Autodesk Inventor part; units mm, degrees
ref_plane "YZ Plane" through (0, 0, 0) normal (1, 0, 0) x (0, 1, 0)
ref_plane "XZ Plane" through (0, 0, 0) normal (0, 1, 0) x (-1, 0, 0)
ref_plane "XY Plane" through (0, 0, 0) normal (0, 0, 1) x (1, 0, 0)
sketch "スケッチ1" plane through (0, 0, 0) normal (0, 0, 1) x (1, 0, 0)
  line L0 (-25, -20) -> (25, -20)
  line L1 (25, -20) -> (25, 20)
  line L2 (25, 20) -> (-25, 20)
  line L3 (-25, 20) -> (-25, -20)
  line L4 (-25, -20) -> (25, 20) construction
  line L5 (25, -20) -> (-25, 20) construction
  line L6 (-22, -17) -> (22, -17) construction
  line L7 (22, -17) -> (22, 17) construction
  line L8 (22, 17) -> (-22, 17) construction
  line L9 (-22, 17) -> (-22, -17) construction
  line L10 (-22, -17) -> (22, 17) construction
  line L11 (22, -17) -> (-22, 17) construction
  circle A0 centre (-22, -17) radius 1.6
  circle A1 centre (-22, 17) radius 1.6
  circle A2 centre (22, -17) radius 1.6
  circle A3 centre (22, 17) radius 1.6
  line L12 (-25, -13.5025) -> (-13.5, -13.5025)
  line L13 (-13.5, -13.5025) -> (-13.5, -1.1025)
  line L14 (-13.5, -1.1025) -> (-25, -1.1025)
  line L15 (-6.2, -20) -> (-6.2, -8.5)
  line L16 (-6.2, -8.5) -> (6.2, -8.5)
  line L17 (6.2, -8.5) -> (6.2, -20)
  line L18 (-25, 0) -> (25, 0) construction
  line L19 (0, -20) -> (0, 20) construction
  line L20 (-25, 13.5025) -> (-13.5, 13.5025)
  line L21 (-13.5, 13.5025) -> (-13.5, 1.1025)
  line L22 (-13.5, 1.1025) -> (-25, 1.1025)
  line L23 (25, -13.5025) -> (13.5, -13.5025)
  line L24 (13.5, -13.5025) -> (13.5, -1.1025)
  line L25 (13.5, -1.1025) -> (25, -1.1025)
  line L26 (13.5, 1.1025) -> (25, 1.1025)
  line L27 (13.5, 13.5025) -> (13.5, 1.1025)
  line L28 (25, 13.5025) -> (13.5, 13.5025)
  line L29 (-8.75, -5.76) -> (8.75, -5.76)
  line L30 (8.75, -5.76) -> (8.75, 15.24)
  line L31 (8.75, 15.24) -> (-8.75, 15.24)
  line L32 (-8.75, 15.24) -> (-8.75, -5.76)
  line L33 (-8.75, -5.76) -> (8.75, 15.24) construction
  line L34 (8.75, -5.76) -> (-8.75, 15.24) construction
  line L35 (-4.5, 15.24) -> (-4.5, 16.664)
  line L36 (-4.5, 16.664) -> (4.5, 16.664)
  line L37 (4.5, 16.664) -> (4.5, 15.24)
  point P0 (0, 0)
  point P1 (-13.5, -7.3025)
  point P2 (0, -8.5)
  point P3 (0, 4.74)
  point P4 (0, 16.664)
  point P5 (0, 4.74)
  dimension "d0" = 50
  dimension "d1" = 40
  dimension "d2" = 44
  dimension "d3" = 34
  dimension "d4" = 3.2
  dimension "d5" = 3.2
  dimension "d6" = 3.2
  dimension "d7" = 3.2
  dimension "d8" = 11.5
  dimension "d9" = 12.4
  dimension "d10" = 7.3025
  dimension "d11" = 11.5
  dimension "d12" = 12.4
  dimension "d17" = 17.5
  dimension "d18" = 21
  dimension "d19" = 9
  dimension "d20" = 1.424
  dimension "d21" = 15.26
extrude "押し出し1" add sketch "スケッチ1" along normal blind 1.6 contours L3 L12 L13 L14 L22 L21 L20 L2 L1 L28 L27 L26 L25 L24 L23 L0 L17 L16 L15 | L15 L16 L17 L0 | L3 L14 L13 L12 | L3 L20 L21 L22 | L23 L24 L25 L1 | L26 L27 L28 L1 | L32 L31 L30 L29 | L35 L36 L37 L31
extrude "押し出し2" add sketch "スケッチ1" along normal blind 7.7 contours L15 L16 L17 L0 | L3 L14 L13 L12 | L3 L20 L21 L22 | L23 L24 L25 L1 | L26 L27 L28 L1
extrude "押し出し3" add sketch "スケッチ1" along normal blind 9.34 contours L32 L31 L30 L29 | L35 L36 L37 L31
equation "\"d5\" = d4"
equation "\"d6\" = d4"
equation "\"d7\" = d4"
equation "\"d11\" = d8"
equation "\"d12\" = d9"
properties part number "Quad-Load-Cell-Amplifier-to-RS-485-Conv-Module"
Check sheet for the modelled part. Datum: model origin and axes. Units: mm. A direction names the side the tool comes from. Round coordinates to 2 decimals unless told otherwise and drop trailing zeros. Loops run counter-clockwise (first coordinate to the right, second up) from the corner with the lowest first, then second, coordinate; pieces in that order, holes last. Notation, with made-up numbers: M -4.5,-17.75 L 23.5,-17.75 A23 ccw 23.5,4.25 Z; hole C 35.25,81 d4. An arc over 180 degrees is marked long. One line per question, with ' | ' between items. Start each with the question number.
Item 1: Section check A-A (y = -17). Record the boundary of the cut face in (x, z).
Item 2: Section check B-B (z = 5.25). Record the boundary of the cut face in (x, y).
Item 3: Scan lines: probe 1 along Y at (x, z) = (22, 0.6); probe 2 along X at (y, z) = (-11, 6); probe 3 along Y at (x, z) = (17.5, 7). Record each from-to range of solid material in increasing order.
Item 4: Set-up check for faces 3 (the face through (-13.5, -7, 5)), 4 (the face through (19, 13.502, 5)), 5 (the face through (-19, 7, 7.7)): record each of +Z, -Z, +X, -X, +Y, -Y from which the full face is reachable in a straight line by a thin tool's end or side.
Item 5: Section check D-D (x = -0.5). Record the boundary of the cut face in (y, z).
Item 6: Section check C-C (x = 22). Record the boundary of the cut face in (y, z).
Item 7: Release check for a two-part mould opening along X. For faces 1 (the face through (-19, -7, 7.7)), 2 (the face through (21.792, 15.414, 0.789)) record: released by +X, released by -X, zero draft, split by the parting line, or undercut.
Item 8: Gauge pin test, flat ends, axial feed: pin 1 Ø1.3 at (x, z) = (-6, 5.5) entering from +Y; pin 2 Ø3 at (x, y) = (-22, -17) entering from -Z; pin 3 Ø6 at (x, y) = (1, -10) entering from +Z; pin 4 Ø5 at (x, y) = (-22, 17) entering from +Z. Record the tip position at first contact, or that the pin passes through.
Worked out:
1) outline: M -25,0 L -23.6,0 L -23.6,1.6 L -25,1.6 Z; M -20.4,0 L 20.4,0 L 20.4,1.6 L 6.2,1.6 L 6.2,7.7 L -6.2,7.7 L -6.2,1.6 L -20.4,1.6 Z; M 23.6,0 L 25,0 L 25,1.6 L 23.6,1.6 Z
2) outline: M -25,-13.5 L -13.5,-13.5 L -13.5,-1.1 L -25,-1.1 Z; M -25,1.1 L -13.5,1.1 L -13.5,13.5 L -25,13.5 Z; M -8.75,-5.76 L 8.75,-5.76 L 8.75,15.24 L 4.5,15.24 L 4.5,16.66 L -4.5,16.66 L -4.5,15.24 L -8.75,15.24 Z; M -6.2,-20 L 6.2,-20 L 6.2,-8.5 L -6.2,-8.5 Z; M 13.5,-13.5 L 25,-13.5 L 25,-1.1 L 13.5,-1.1 Z; M 13.5,1.1 L 25,1.1 L 25,13.5 L 13.5,13.5 Z
3) probe 1: -20 to -18.6, -15.4 to 15.4, 18.6 to 20 | probe 2: -25 to -13.5, -6.2 to 6.2, 13.5 to 25 | probe 3: -13.5 to -1.1, 1.1 to 13.5
4) face 3: +Z, +Y, -Y | face 4: +Z, +X, +Y | face 5: +Z, -X, +Y, -Y
5) outline: M -20,0 L 20,0 L 20,1.6 L 16.66,1.6 L 16.66,9.34 L -5.76,9.34 L -5.76,1.6 L -8.5,1.6 L -8.5,7.7 L -20,7.7 Z
6) outline: M -20,0 L -18.6,0 L -18.6,1.6 L -20,1.6 Z; M -15.4,0 L 15.4,0 L 15.4,1.6 L 13.5,1.6 L 13.5,7.7 L 1.1,7.7 L 1.1,1.6 L -1.1,1.6 L -1.1,7.7 L -13.5,7.7 L -13.5,1.6 L -15.4,1.6 Z; M 18.6,0 L 20,0 L 20,1.6 L 18.6,1.6 Z
7) face 1: zero draft | face 2: undercut
8) pin 1: y = 15.24 | pin 2: through | pin 3: z = 7.7 | pin 4: z = 1.6
